The model under review builds one solid part; all positions refer to its coordinate system, in mm. A direction names the side the tool comes from. Round coordinates to 2 decimals unless told otherwise and drop trailing zeros. Write each loop counter-clockwise with the first axis right and the second up, starting at its lowest first coordinate (ties: lowest second). Pieces come first, ordered by that corner, then holes. Notation, with made-up numbers: M 20.5,60 L 52.5,60 A27 ccw 52.5,93 Z; hole C 51,19 d8. An arc over 180 degrees is marked long. One line per item, written item: value. Start each with the question number.
1) Take a section at A-A, the plane y = 25. Write out the cut boundary in (x, z).
2) Take a section at D-D, the plane x = 6.25. State how many separate pieces and enclosed holes the cut face has, and give its area (3 significant figures).
3) For P1, Ø1.5, axis at x = 3.5, z = 4, coming from the -Y side; P2, Ø0.6, axis at x = 0, y = 33, coming from the +Z side; P3, Ø2, axis at y = 12, z = 7.5, coming from the +X side, all flat-tipped, find the tip position at first contact; note any pin that passes through.
4) Tool access review of faces 1 (the face through (0.8, 11.7, 7.8)), 2 (the face through (0.285, 24.843, 0.301)), 3 (the face through (0.39, 11.15, 5.31)): name each direction out of +Z, -Z, +X, -X, +Y, -Y from which nothing blocks a thin tool from reaching the whole face with its end or side.
5) Wall thickness on probe 1 along Z at (x, y) = (10.25, 19); probe 2 along Y at (x, z) = (6.25, 1.25); probe 3 along Y at (x, z) = (6.25, 0.5): over which ranges is each line inside the solid? List them lowest first.
6) Take a section at C-C, the plane y = 18. Write out the cut boundary in (x, z).
7) Take a section at B-B, the plane z = 5.4. Write out the cut boundary in (x, y).
8) Mouldability with a two-part tool opening along Z and no side actions: class faces 4 (the face through (5.87, 47.29, 10.16)), 5 (the face through (6, 23, 1.3)), 6 (the face through (12.215, 24.157, 10.499)) as +Z half, -Z half, draft (parallel to the pull), parting line (faces both ways), or undercut.
from build123d import *

# Parameters (mm, degrees)
BASE_EXTRUSION_DEPTH    = 10.8
CONG_1_R                = 1
CONG_2_R                = 1
ESQUISSE2_W             = 8.2
ESQUISSE2_H             = 65.100918748
ENL_V_MAT_EXTRU_1_DEPTH = 11.7
ESQUISSE3_W             = 8.2
ESQUISSE3_H             = 9.8
ENL_V_MAT_EXTRU_3_DEPTH = 11.7
ESQUISSE4_R             = 2
ESQUISSE4_R_2           = 1.75
ENL_V_MAT_EXTRU_4_DEPTH = 58.666736534


with BuildPart() as part:
    # Esquisse1 → Base-Extrusion (new body)
    with BuildSketch(Plane.XY):
        with BuildLine():
            Line((0, 0), (0, 49))
            ThreePointArc((0, 49), (6.25, 55.25), (12.5, 49))
            Line((12.5, 49), (12.5, 0))
            ThreePointArc((12.5, 0), (6.25, -6.25), (0, 0))
        make_face()
    extrude(amount=BASE_EXTRUSION_DEPTH)

    # Congé1
    cong_1_edges = [part.edges().sort_by_distance(p)[0] for p in [
        (6.25, 55.25, 10.8),
        (0, 24.5, 10.8),
        (6.25, -6.25, 10.8),
        (12.5, 24.5, 10.8),
    ]]
    fillet(cong_1_edges, radius=CONG_1_R)

    # Congé2
    cong_2_edges = [part.edges().sort_by_distance(p)[0] for p in [
        (0, 24.5, 0),
        (6.25, 55.25, 0),
        (12.5, 24.5, 0),
        (6.25, -6.25, 0),
    ]]
    fillet(cong_2_edges, radius=CONG_2_R)

    # Esquisse2 → Enlèv. mat.-Extru.1 (cut)
    with BuildSketch(Plane(origin=(12.5, 0, 0), x_dir=(0, 0, -1), z_dir=(1, 0, 0))):
        with Locations((-5.4, 21.424016652)):
            Rectangle(ESQUISSE2_W, ESQUISSE2_H)
    extrude(amount=-ENL_V_MAT_EXTRU_1_DEPTH, mode=Mode.SUBTRACT)

    # Esquisse3 → Enlèv. mat.-Extru.3 (cut)
    with BuildSketch(Plane.ZY):
        with BuildLine():
            Line((1.4, 49.948011349), (1.4, 15.15))
            ThreePointArc((1.4, 15.15), (5.4, 11.15), (9.4, 15.15))
            Line((9.4, 15.15), (9.4, 49.948011349))
            Line((9.4, 49.948011349), (1.4, 49.948011349))
        make_face()
        with Locations((5.4, -1.35)):
            Rectangle(ESQUISSE3_W, ESQUISSE3_H)
    extrude(amount=-ENL_V_MAT_EXTRU_3_DEPTH, mode=Mode.SUBTRACT)

    # Esquisse4 → Enlèv. mat.-Extru.4 (cut, through all)
    with BuildSketch(Plane.XY.offset(10.8)):
        with Locations((6.25, 0)):
            Circle(ESQUISSE4_R)
        with Locations((6.25, 49)):
            Circle(ESQUISSE4_R_2)
        with Locations((6.25, 18)):
            Circle(ESQUISSE4_R_2)
    extrude(amount=-ENL_V_MAT_EXTRU_4_DEPTH, mode=Mode.SUBTRACT)


solid = part.part
Checked values:
1. outline: M 0,1 A1 ccw 1,0 L 11.5,0 A1 ccw 12.5,1 L 12.5,1.3 L 0.8,1.3 L 0.8,1.4 L 0,1.4 Z; M 0,9.4 L 0.8,9.4 L 0.8,9.5 L 12.5,9.5 L 12.5,9.8 A1 ccw 11.5,10.8 L 1,10.8 A1 ccw 0,9.8 Z
2. separate pieces: 7
2. enclosed holes: 0
2. area: 141 mm2
3. P1: stops at y = 53.97
3. P2: stops at z = 10.51
3. P3: stops at x = 0.8
4. face 1: +X, +Y, -Y
4. face 2: -Z, -X, +Y, -Y
4. face 3: +X, -X
5. probe 1: z = 0 to 1.3, 9.5 to 10.8
5. probe 2: y = -6.25 to -2, 2 to 16.25, 19.75 to 47.25, 50.75 to 55.25
5. probe 3: y = -6.12 to -2, 2 to 16.25, 19.75 to 47.25, 50.75 to 55.12
6. outline: M 0,1 A1 ccw 1,0 L 4.5,0 L 4.5,1.3 L 0.8,1.3 L 0.8,1.4 L 0,1.4 Z; M 0,9.4 L 0.8,9.4 L 0.8,9.5 L 4.5,9.5 L 4.5,10.8 L 1,10.8 A1 ccw 0,9.8 Z; M 8,0 L 11.5,0 A1 ccw 12.5,1 L 12.5,1.3 L 8,1.3 Z; M 8,9.5 L 12.5,9.5 L 12.5,9.8 A1 ccw 11.5,10.8 L 8,10.8 Z
7. outline: M 0,3.55 L 0.8,3.55 L 0.8,11.15 L 0,11.15 Z; M 0.07,49.95 L 0.8,49.95 L 0.8,52.06 A6.25 ccw Z; M 2.47,53.97 L 10.03,53.97 A6.25 ccw Z
8. face 4: draft
8. face 5: undercut
8. face 6: +Z half
